Verification items for this drawing (mm, ordinates from the low corner). A direction names the side the tool comes from. Round coordinates to 2 decimals unless told otherwise and drop trailing zeros. Write each loop counter-clockwise with the first axis right and the second up, starting at its lowest first coordinate (ties: lowest second). Pieces come first, ordered by that corner, then holes. Notation, with made-up numbers: M -39.75,65.5 L -20.75,65.5 A16 ccw -20.75,72.5 Z; hole C 0,80 d10. An arc over 180 degrees is marked long. One line per question, with ' | ' between items. Start each with the question number.
Q1. Cross-section at D-D (y = 21.5). Record the boundary of the cut face in (x, z).
Q2. Tool access check on the marked faces 5, 6, 7, 8 and 9. Record the directions out of +Z, -Z, +X, -X, +Y, -Y that give a thin tool (end or side, any length) a straight path to the whole face; none if there is none.
Q3. Cross-section at B-B (y = 11). Record the boundary of the cut face in (x, z).
Q4. Cross-section at A-A (z = 12). Record the boundary of the cut face in (x, y), then the cut area to 3 significant figures.
Q5. Thickness scan on line 1 along Z through (x, y) = (45, 16); line 2 along X through (y, z) = (12.75, 20); line 3 along X through (y, z) = (39, 25). Record the ranges inside material, lowest first. Write a range as from..to.
Q6. Gauge pin test, flat ends, axial feed: pin 1 (12 mm diameter, centred on x = 41, z = 32.5, fed in from -Y); pin 2 (7.5 mm diameter, centred on x = 79, z = 13.5, fed in from +Y); pin 3 (9 mm diameter, centred on y = 33, z = 20.5, fed in from +X). Record the tip position at first contact, or that the pin passes through.
Q7. Release check for a two-part mould opening along Z. For the marked faces 1, 2, 3 and 4 record: released by +Z, released by -Z, zero draft, split by the parting line, or undercut.
Q8. Cross-section at C-C (x = 63.5). Record the boundary of the cut face in (y, z), then the cut area to 3 significant figures.
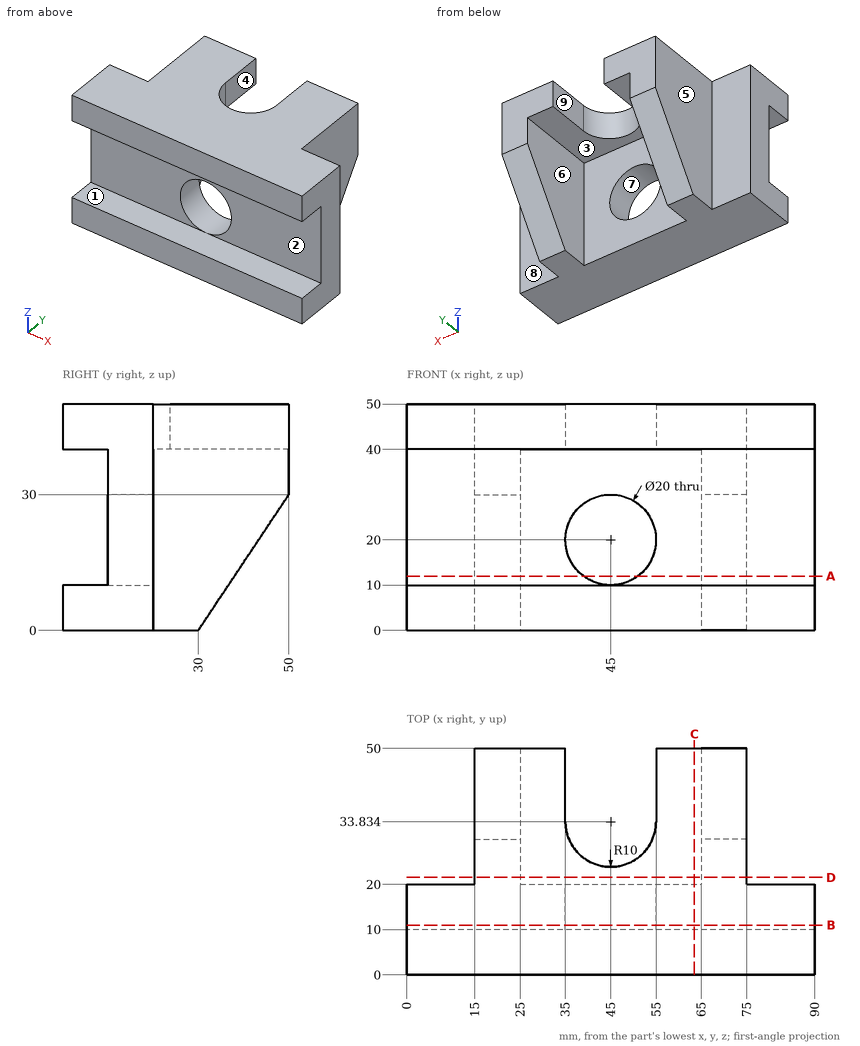
Determined:
1) outline: M 15,0 L 25,0 L 25,40 L 65,40 L 65,0 L 75,0 L 75,50 L 15,50 Z
2) face 5: +Z, -Z, -X, +Y | face 6: -Z, +Y | face 7: +Y, -Y | face 8: +Z, -Z, +X, +Y | face 9: +Z, -Z, +Y
3) outline: M 0,0 L 90,0 L 90,50 L 0,50 Z; hole C 45,20 d20
4) outline: M 0,10 L 39,10 L 39,20 L 25,20 L 25,38 L 15,38 L 15,20 L 0,20 Z; M 51,10 L 90,10 L 90,20 L 75,20 L 75,38 L 65,38 L 65,20 L 51,20 Z | area: 1,140 mm²
5) line 1: z = 0..10, 30..50 | line 2: x = 0..35, 55..90 | line 3: x = 15..25, 65..75
6) pin 1: stops at y = 10 | pin 2: stops at y = 20 | pin 3: stops at x = 75
7) face 1: undercut | face 2: undercut | face 3: released by -Z | face 4: zero draft
8) outline: M 0,0 L 20,0 L 20,40 L 50,40 L 50,50 L 0,50 L 0,40 L 10,40 L 10,10 L 0,10 Z | area: 1,000 mm²
